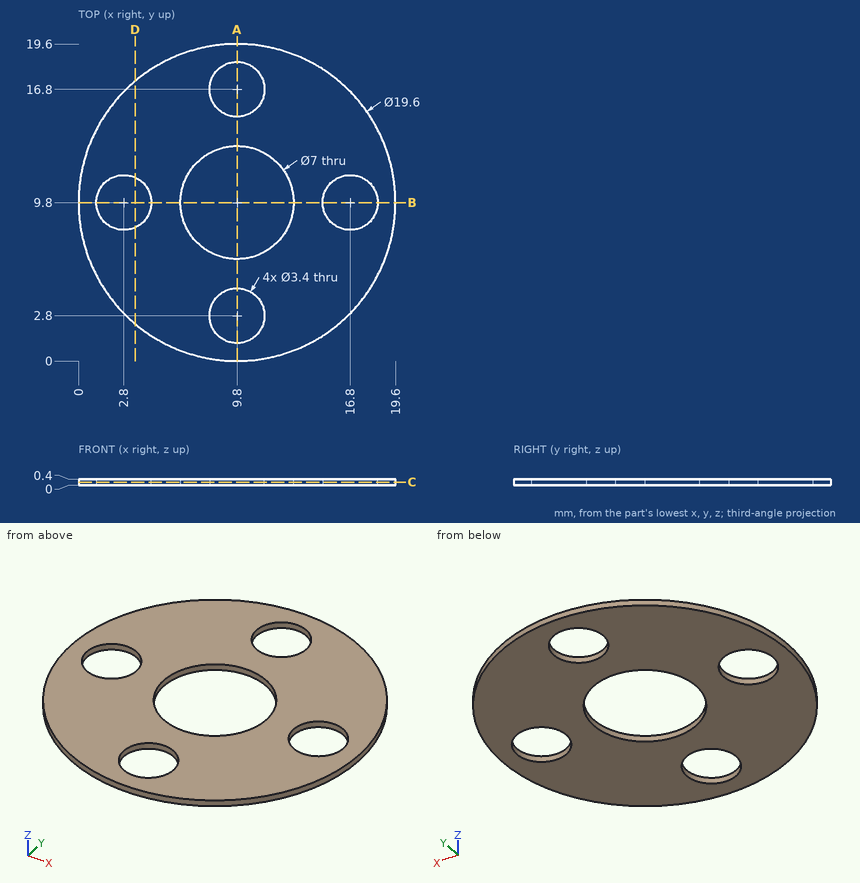
Study the drawing (mm; zero at the part's minimum x, y, z) and answer. Give positions to 0.01 mm unless a question says otherwise; leave off trailing zeros. Write each loop counter-clockwise with the first axis right and the second up, starting at its lowest first coordinate (ties: lowest second). Pieces come first, ordered by that corner, then holes.
(1) The part is cut by section A-A on x = 9.8. Write down the section's boundary in (y, z), plus the area to 3 significant figures.
Final values:
outline: (0, 0) - (1.1, 0) - (1.1, 0.4) - (0, 0.4) - close; (4.5, 0) - (6.3, 0) - (6.3, 0.4) - (4.5, 0.4) - close; (13.3, 0) - (15.1, 0) - (15.1, 0.4) - (13.3, 0.4) - close; (18.5, 0) - (19.6, 0) - (19.6, 0.4) - (18.5, 0.4) - close
area: 2.32 mm2
(2) The part is cut by section D-D on x = 3.5. Write down the section's boundary in (y, z).
Final values:
outline: (2.29, 0) - (8.25, 0) - (8.25, 0.4) - (2.29, 0.4) - close; (11.35, 0) - (17.31, 0) - (17.31, 0.4) - (11.35, 0.4) - close
(3) Straight lines are drawn through the part: line 1 (Y direction, x = 9.8, z = 0.1); line 2 (X direction, y = 10.5, z = 0.1); line 3 (Y direction, x = 8.5, z = 0.35). For each, find the intervals that lie inside material, in ascending order.
Final values:
line 1: y = 0 to 1.1, 4.5 to 6.3, 13.3 to 15.1, 18.5 to 19.6
line 2: x = 0.03 to 1.25, 4.35 to 6.37, 13.23 to 15.25, 18.35 to 19.57
line 3: y = 0.09 to 1.7, 3.9 to 6.55, 13.05 to 15.7, 17.9 to 19.51
(4) The part is cut by section C-C on z = 0.2. Write down the section's boundary in (x, y).
Final values:
outline: circle Ø19.6 at (9.8, 9.8); hole circle Ø3.4 at (2.8, 9.8); hole circle Ø7 at (9.8, 9.8); hole circle Ø3.4 at (9.8, 2.8); hole circle Ø3.4 at (9.8, 16.8); hole circle Ø3.4 at (16.8, 9.8)
